```python
from build123d import *

# Parameters (mm, degrees)
F0_W     = 9.543723
F0_H     = 3
F0_W_2   = 2.456277
F1_DEPTH = 25
F2_R     = 0.65
F3_R     = 1.228
F4_R     = 1


with BuildPart() as f1:
    # F0 (on Top) → F1 (new body)
    with BuildSketch(Plane.XY):
        with Locations((-54.771861, 30)):
            Rectangle(F0_W, F0_H)
        with Locations((-48.771861, 30)):
            Rectangle(F0_W_2, F0_H)
        Polygon((-46.387445, 1), (-47.543723, 31.5), (-47.543723, 28.5), (-50, 28.5), (-50, 0), (-50, -31.5), (-47.543723, -31.5), (-46.387445, -1), (-40.370852, -1), (-40.357002, -1.365324), (-36.780361, -1.581997), (-36.758297, -1), (-30.741703, -1), (-30.705688, -1.95), (-27.173276, -2.163993), (-27.129148, -1), (-21.112555, -1), (-21.054374, -2.534676), (-17.5, -2.75), (0, -2.75), (17.5, -2.75), (21.054374, -2.534676), (21.112555, -1), (27.129148, -1), (27.173276, -2.163993), (30.705688, -1.95), (30.741703, -1), (36.758297, -1), (36.780361, -1.581997), (40.357002, -1.365324), (40.370852, -1), (46.387445, -1), (47.543723, -31.5), (50, -31.5), (50, 0), (50, 28.5), (47.543723, 28.5), (47.543723, 31.5), (46.387445, 1), (40.370852, 1), (40.357002, 1.365324), (36.780361, 1.581997), (36.758297, 1), (30.741703, 1), (30.705688, 1.95), (27.173276, 2.163993), (27.129148, 1), (21.112555, 1), (21.054374, 2.534676), (17.5, 2.75), (0, 2.75), (-17.5, 2.75), (-21.054374, 2.534676), (-21.112555, 1), (-27.129148, 1), (-27.173276, 2.163993), (-30.705688, 1.95), (-30.741703, 1), (-36.758297, 1), (-36.780361, 1.581997), (-40.357002, 1.365324), (-40.370852, 1), align=None)
        Polygon((-36.780361, -1.581997), (-40.357002, -1.365324), (-39.214574, -31.5), (-37.914574, -31.5), align=None)
        Polygon((-39.214574, 31.5), (-40.357002, 1.365324), (-36.780361, 1.581997), (-37.914574, 31.5), align=None)
        Polygon((-27.173276, -2.163993), (-30.705688, -1.95), (-29.585426, -31.5), (-28.285426, -31.5), align=None)
        Polygon((-29.585426, 31.5), (-30.705688, 1.95), (-27.173276, 2.163993), (-28.285426, 31.5), align=None)
        Polygon((-17.5, -2.75), (-21.054374, -2.534676), (-19.956277, -31.5), (-18.656277, -31.5), align=None)
        Polygon((-19.956277, 31.5), (-21.054374, 2.534676), (-17.5, 2.75), (-18.656277, 31.5), align=None)
        Polygon((21.054374, -2.534676), (17.5, -2.75), (18.656277, -31.5), (19.956277, -31.5), align=None)
        Polygon((18.656277, 31.5), (17.5, 2.75), (21.054374, 2.534676), (19.956277, 31.5), align=None)
        Polygon((28.285426, 31.5), (27.173276, 2.163993), (30.705688, 1.95), (29.585426, 31.5), align=None)
        Polygon((30.705688, -1.95), (27.173276, -2.163993), (28.285426, -31.5), (29.585426, -31.5), align=None)
        Polygon((40.357002, -1.365324), (36.780361, -1.581997), (37.914574, -31.5), (39.214574, -31.5), align=None)
        Polygon((37.914574, 31.5), (36.780361, 1.581997), (40.357002, 1.365324), (39.214574, 31.5), align=None)
        with Locations((54.771861, 30)):
            Rectangle(F0_W, F0_H)
        with Locations((48.771861, 30)):
            Rectangle(F0_W_2, F0_H)
        Polygon((-36.758297, -1), (-36.780361, -1.581997), (-30.705688, -1.95), (-30.741703, -1), align=None)
        Polygon((-27.129148, -1), (-27.173276, -2.163993), (-21.054374, -2.534676), (-21.112555, -1), align=None)
        Polygon((-21.054374, 2.534676), (-27.173276, 2.163993), (-27.129148, 1), (-21.112555, 1), align=None)
        Polygon((-30.705688, 1.95), (-36.780361, 1.581997), (-36.758297, 1), (-30.741703, 1), align=None)
        Polygon((-40.357002, 1.365324), (-46.387445, 1), (-40.370852, 1), align=None)
        Polygon((-40.370852, -1), (-46.387445, -1), (-40.357002, -1.365324), align=None)
        Polygon((21.112555, -1), (21.054374, -2.534676), (27.173276, -2.163993), (27.129148, -1), align=None)
        Polygon((27.173276, 2.163993), (21.054374, 2.534676), (21.112555, 1), (27.129148, 1), align=None)
        Polygon((36.780361, 1.581997), (30.705688, 1.95), (30.741703, 1), (36.758297, 1), align=None)
        Polygon((30.741703, -1), (30.705688, -1.95), (36.780361, -1.581997), (36.758297, -1), align=None)
        Polygon((40.370852, -1), (40.357002, -1.365324), (46.387445, -1), align=None)
        Polygon((46.387445, 1), (40.357002, 1.365324), (40.370852, 1), align=None)
    extrude(amount=F1_DEPTH)

    # F2
    f2_edges = [f1.edges().sort_by_distance(p)[0] for p in [
        (29.585426, 31.5, 12.5),
        (28.285426, 31.5, 12.5),
        (39.214574, 31.5, 12.5),
        (37.914574, 31.5, 12.5),
        (19.956277, 31.5, 12.5),
        (18.656277, 31.5, 12.5),
        (-18.656277, 31.5, 12.5),
        (-19.956277, 31.5, 12.5),
        (-28.285426, 31.5, 12.5),
        (-29.585426, 31.5, 12.5),
        (-37.914574, 31.5, 12.5),
        (-39.214574, 31.5, 12.5),
        (-39.214574, -31.5, 12.5),
        (-37.914574, -31.5, 12.5),
        (-29.585426, -31.5, 12.5),
        (-28.285426, -31.5, 12.5),
        (-19.956277, -31.5, 12.5),
        (-18.656277, -31.5, 12.5),
        (18.656277, -31.5, 12.5),
        (19.956277, -31.5, 12.5),
        (28.285426, -31.5, 12.5),
        (29.585426, -31.5, 12.5),
        (37.914574, -31.5, 12.5),
        (39.214574, -31.5, 12.5),
    ]]
    fillet(f2_edges, radius=F2_R)

    # F3
    f3_edges = [f1.edges().sort_by_distance(p)[0] for p in [
        (-50, -31.5, 12.5),
        (-47.543723, -31.5, 12.5),
        (47.543723, -31.5, 12.5),
        (50, -31.5, 12.5),
        (-47.543723, 31.5, 12.5),
        (47.543723, 31.5, 12.5),
    ]]
    fillet(f3_edges, radius=F3_R)

    # F4
    f4_edges = [f1.edges().sort_by_distance(p)[0] for p in [
        (-50, 28.5, 12.5),
        (-40.357002, 1.365324, 12.5),
        (-46.387445, 1, 12.5),
        (-36.780361, 1.581997, 12.5),
        (-30.705688, 1.95, 12.5),
        (-21.054374, 2.534676, 12.5),
        (-27.173276, 2.163993, 12.5),
        (-40.357002, -1.365324, 12.5),
        (-46.387445, -1, 12.5),
        (-30.705688, -1.95, 12.5),
        (-21.054374, -2.534676, 12.5),
        (-27.173276, -2.163993, 12.5),
        (-36.780361, -1.581997, 12.5),
        (-17.5, 2.75, 12.5),
        (-17.5, -2.75, 12.5),
        (17.5, -2.75, 12.5),
        (17.5, 2.75, 12.5),
        (27.173276, 2.163993, 12.5),
        (27.173276, -2.163993, 12.5),
        (36.780361, -1.581997, 12.5),
        (30.705688, -1.95, 12.5),
        (30.705688, 1.95, 12.5),
        (36.780361, 1.581997, 12.5),
        (40.357002, -1.365324, 12.5),
        (40.357002, 1.365324, 12.5),
        (46.387445, 1, 12.5),
        (46.387445, -1, 12.5),
        (-59.543723, 31.5, 12.5),
        (-59.543723, 28.5, 12.5),
        (59.543723, 31.5, 12.5),
        (59.543723, 28.5, 12.5),
        (21.054374, 2.534676, 12.5),
        (21.054374, -2.534676, 12.5),
    ]]
    fillet(f4_edges, radius=F4_R)


solid = f1.part
```
Model file for the job. Use its own axes, mm. A direction names the side the tool comes from. Give positions to 0.01 mm unless a question says otherwise; leave off trailing zeros. Order: outer loops, then holes, each group sorted by start corner. A loop starts at its lowest first (then second) coordinate and runs counter-clockwise, first axis right, second up.
1) 3-axis set-ups, long thin cutter, end or side, ignore diameter. For faces 4 (the flat face through (-39.773, 16.773, 12.325)), 5 (the flat face through (27.73, -16.84, 12.32)): which of +Z, -Z, +X, -X, +Y, -Y reach the whole face in a straight line?
2) Saw through at C-C, the plane x = 34. Write the cut outline in (y, z), then the cut area to 3 significant figures.
3) Mould opens along X. For faces 1 (the flat face through (4, 0, 0)), 2 (the flat face through (50, -1, 12)), 3 (the flat face through (43.285, -1.188, 12.325)) say: +X half, -X half, draft (parallel to the pull), parting line (faces both ways), or undercut.
4) Pin check, flat tips, straight feed: pin 1 (4.5 mm diameter, centred on x = 53, z = 9, fed in from -Y); pin 2 (4 mm diameter, centred on y = 4.5, z = 12.5, fed in from -X); pin 3 (1.5 mm diameter, centred on x = 31.5, y = -11.5, fed in from +Z); pin 4 (10 mm diameter, centred on y = -1.5, z = 3.5, fed in from +X). Stop position of each tip, or through.
5) Wall check: probe 1 along Y at (x, z) = (29, 19.75); probe 2 along Y at (x, z) = (-26, 1.75). Give the ranges that are in metal, low to high.
6) Saw through at A-A, the plane y = -21.5. Count the separate pieces of the cut face and the enclosed holes in it, then the cut area to 3 significant figures.
Computed:
1. face 4: +Z, -Z, +Y
1. face 5: +Z, -Z, -Y
2. outline: (-1.75, 0) - (1.75, 0) - (1.75, 25) - (-1.75, 25) - close
2. area: 87.5 mm2
3. face 1: draft
3. face 2: +X half
3. face 3: undercut
4. pin 1: stops at y = 28.5
4. pin 2: stops at x = -50
4. pin 3: passes through
4. pin 4: stops at x = 50
5. probe 1: y = -31.5 to 31.5
5. probe 2: y = -2.24 to 2.24
6. separate pieces: 8
6. enclosed holes: 0
6. area: 452 mm2
